Could you check a few things on this model? Use its own coordinates, in mm. A direction names the side the tool comes from. Coordinates: 2 decimals unless noted, no trailing zeros. Order: outer loops, then holes, each group sorted by start corner. A loop starts at its lowest first (then second) coordinate and runs counter-clockwise, first axis right, second up. Notation, with made-up numbers: M -28,4 L -3,4 A18 ccw -3,34 Z; hole C 27.5,18 d9. An arc over 180 degrees is marked long. One line per question, with ' | ' between items. Start each with the question number.
from build123d import *

# Parameters (mm, degrees)
F0_R     = 8
F1_DEPTH = 5


with BuildPart() as f1:
    # F0 (on Top) → F1 (new body)
    with BuildSketch(Plane.XY):
        with BuildLine():
            ThreePointArc((-7.472874, 17.144103), (4.536123, 26.589658), (0, 12))
            ThreePointArc((0, 12), (-6.844348, 9.856719), (-11.243802, 4.192483))
            ThreePointArc((-11.243802, 4.192483), (-13.258407, 1.712126), (-16.363653, 0.958304))
            ThreePointArc((-16.363653, 0.958304), (-27.448872, -14.291414), (-8.782148, -16.935157))
            ThreePointArc((-8.782148, -16.935157), (-8.471386, -15.717191), (-9.19647, -14.690416))
            ThreePointArc((-9.19647, -14.690416), (-10.218732, -14.51437), (-11.110792, -15.043751))
            ThreePointArc((-11.110792, -15.043751), (-25.295381, -9.366431), (-10.392305, -6))
            ThreePointArc((-10.392305, -6), (-5.113995, -10.855739), (1.991104, -11.83366))
            ThreePointArc((1.991104, -11.83366), (5.146458, -12.33818), (7.351911, -14.650492))
            ThreePointArc((7.351911, -14.650492), (26.101164, -16.625714), (19.05735, 0.862015))
            ThreePointArc((19.05735, 0.862015), (17.84718, 0.52216), (17.320508, -0.619168))
            ThreePointArc((17.320508, -0.619168), (17.679179, -1.592497), (18.583666, -2.100352))
            ThreePointArc((18.583666, -2.100352), (20.759257, -17.223227), (10.392305, -6))
            ThreePointArc((10.392305, -6), (11.958343, 0.99902), (9.252698, 7.641176))
            ThreePointArc((9.252698, 7.641176), (8.111948, 10.626054), (9.011742, 13.692188))
            ThreePointArc((9.011742, 13.692188), (1.347709, 30.917128), (-10.275202, 16.073142))
            ThreePointArc((-10.275202, 16.073142), (-9.375794, 15.195031), (-8.124038, 15.309584))
            ThreePointArc((-8.124038, 15.309584), (-7.460447, 16.106867), (-7.472874, 17.144103))
        make_face()
        Circle(F0_R, mode=Mode.SUBTRACT)
    extrude(amount=F1_DEPTH)


solid = f1.part
(1) We'd pull the mould along Y, two halves only. Please class faces 1 (the cylindrical face through (8.114, 10.581, 2.465)), 2 (the cylindrical face through (25.907, -16.876, 2.465)), 3 (the cylindrical face through (-13.22, 1.737, 2.465)), 4 (the flat face through (-0.1, -8.4, 5)): +Y half, -Y half, draft (parallel to the pull), parting line (faces both ways), or undercut.
(2) For P1, Ø14.5, axis at x = 0, y = 0, coming from the -Z side; P2, Ø1, axis at x = 13, z = 3, coming from the +Y side; P3, Ø2, axis at x = -4, z = 3, coming from the +Y side; P4, Ø1.5, axis at x = -22, z = 2, coming from the +Y side, each with a flat end and sliding along its axis, tell me the tip position at first contact or that it passes through.
(3) Imagine slicing it at A-A, the plane y = 0. Write out the boundary of the cut face in (x, z), plus the area to 3 significant figures.
(4) Imagine slicing it at D-D, the plane z = 3.3. Write out the boundary of the cut face in (x, y) (1 decimal).
(5) On a 3-axis mill with a long thin cutter (end or side, diameter ignored), from which of +Z, -Z, +X, -X, +Y, -Y can I reach the whole of each face in a straight line? I mean faces 5 (the cylindrical face through (11.966, 0.897, 2.465)), 6 (the cylindrical face through (-6.76, 9.915, 2.465)), 7 (the cylindrical face through (5.11, -12.32, 2.46)). Say none if no direction works.
(6) Imagine slicing it at B-B, the plane y = 20. Write out the boundary of the cut face in (x, z).
(7) If I drill on line 1 along Y through (x, z) = (0, 1.8); line 2 along X through (y, z) = (20, 0.95); line 3 along X through (y, z) = (-10, 1.35), over which ranges is the centre line in solid material (lowest first)? Write a range as from..to.
(8) Imagine slicing it at C-C, the plane x = 1. Write out the boundary of the cut face in (y, z).
Answers:
1) face 1: undercut | face 2: parting line | face 3: +Y half | face 4: draft
2) P1: through | P2: y = -16.38 | P3: y = 30.58 | P4: y = 0.27
3) outline: M -21.9,0 L -8,0 L -8,5 L -21.9,5 Z; M 8,0 L 12,0 L 12,5 L 8,5 Z; M 17.45,0 L 21.9,0 L 21.9,5 L 17.45,5 Z | area: 112 mm²
4) outline: M -16.4,1 A11 ccw long -8.8,-16.9 A1.5 ccw -11.1,-15 A8 cw long -10.4,-6 A12 ccw 2,-11.8 A5 cw 7.4,-14.7 A11 ccw long 19.1,0.9 A1.5 ccw 17.3,-0.6 A1.5 ccw 18.6,-2.1 A8 cw long 10.4,-6 A12 ccw 9.3,7.6 A5 cw 9,13.7 A11 ccw long -10.3,16.1 A1.5 ccw -8.1,15.3 A1.5 ccw -7.5,17.1 A8 cw long 0,12 A12 ccw -11.2,4.2 A5 cw Z; hole C 0,0 d16
5) face 5: +Z, -Z | face 6: +Z, -Z, -X | face 7: +Z, -Z, -Y
6) outline: M -11,0 L -8,0 L -8,5 L -11,5 Z; M 8,0 L 11,0 L 11,5 L 8,5 Z
7) line 1: -12..-8, 8..12, 28..31 | line 2: -11..-8, 8..11 | line 3: -28.32..-25.32, -6.63..9.32, 25.32..28.32
8) outline: M -11.96,0 L -7.94,0 L -7.94,5 L -11.96,5 Z; M 7.94,0 L 12.06,0 L 12.06,5 L 7.94,5 Z; M 27.94,0 L 30.95,0 L 30.95,5 L 27.94,5 Z
